from build123d import *

# Parameters (mm, degrees)
SKETCH_1_W               = 20
SKETCH_1_H               = 10
EXTRUDE_1_DEPTH          = 8.5
EXTRUDE_3_DEPTH          = 8.5
EXTRUDE_3_DEPTH_BACK     = 13
CUT_EXTRUDE_1_DEPTH      = 9
SKETCH_11_W              = 7.4
SKETCH_11_H              = 18
EXTRUDE_5_DEPTH          = 0.4
SKETCH_14_W              = 13
SKETCH_14_H              = 8.5
CUT_EXTRUDE_7_DEPTH      = 8
SKETCH_6_R               = 1.75
CUT_EXTRUDE_2_DEPTH      = 12.8
CUT_EXTRUDE_3_DEPTH      = 35.441980199
CUT_EXTRUDE_3_DEPTH_BACK = 12.9
SKETCH_15_W              = 3.5
SKETCH_15_H              = 8
CUT_EXTRUDE_8_DEPTH      = 8.5
SKETCH_12_R              = 1.6
CUT_EXTRUDE_4_DEPTH      = 35.693082884
SKETCH_13_R              = 3
CUT_EXTRUDE_5_DEPTH      = 4.5
FILLET_1_R               = 2.5
FILLET_2_R               = 4


# Some blends are built 0.0001 mm under size
with BuildPart() as part:
    # Эскиз1 → Бобышка-Вытянуть1 (new body)
    with BuildSketch(Plane.XY):
        with Locations((10, -5)):
            Rectangle(SKETCH_1_W, SKETCH_1_H)
    extrude(amount=EXTRUDE_1_DEPTH)

    # Эскиз4 → Бобышка-Вытянуть3 (add, two sides: drawn at the far end of the back side and taken through both)
    with BuildSketch(Plane(origin=(0, 0, 8.5), x_dir=(-1, 0, 0), z_dir=(0, 0, -1)).offset(-EXTRUDE_3_DEPTH_BACK)):
        with BuildLine():
            Line((4.25, -10), (0, -10))
            Line((0, -10), (0, 0))
            Line((0, 0), (-20, 0))
            Line((-20, 0), (-20, -10))
            Line((-20, -10), (-19.25, -10))
            Line((-19.25, -10), (-19.25, -14))
            ThreePointArc((-19.25, -14), (-18.078427125, -16.828427125), (-15.25, -18))
            Line((-15.25, -18), (4.25, -18))
            ThreePointArc((4.25, -18), (8.25, -14), (4.25, -10))
        make_face()
    extrude(amount=EXTRUDE_3_DEPTH + EXTRUDE_3_DEPTH_BACK)

    # Эскиз5 → Вырез-Вытянуть1 (cut)
    with BuildSketch(Plane.XY.offset(21.5)):
        Polygon((-1.25, -10), (-1.25, -18), (12.25, -18), (12.25, -10), (20, -10), (20, 0), (0, 0), (0, -10), align=None)
    extrude(amount=-CUT_EXTRUDE_1_DEPTH, mode=Mode.SUBTRACT)

    # Эскиз11 → Бобышка-Вытянуть5 (add)
    with BuildSketch(Plane(origin=(0, 0, 0), x_dir=(-1, 0, 0), z_dir=(0, 0, -1))):
        with Locations((-10, -9)):
            Rectangle(SKETCH_11_W, SKETCH_11_H)
    extrude(amount=EXTRUDE_5_DEPTH)

    # Эскиз14 → Вырез-Вытянуть7 (cut)
    with BuildSketch(Plane(origin=(9.75, -18, 0), x_dir=(-1, 0, 0), z_dir=(0, 1, 0))):
        with Locations((19.75, 4.25)):
            Rectangle(SKETCH_14_W, SKETCH_14_H)
    extrude(amount=CUT_EXTRUDE_7_DEPTH, mode=Mode.SUBTRACT)

    # Эскиз6 → Вырез-Вытянуть2 (cut)
    with BuildSketch(Plane.XY.offset(21.5)):
        with Locations((-4.25, -14)):
            Circle(SKETCH_6_R)
        with Locations((15.25, -14)):
            Circle(SKETCH_6_R)
    extrude(amount=-CUT_EXTRUDE_2_DEPTH, mode=Mode.SUBTRACT)

    # Эскиз7 → Вырез-Вытянуть3 (cut, two sides: drawn at the far end of the back side and taken through both)
    with BuildSketch(Plane(origin=(0, 0, 0), x_dir=(-1, 0, 0), z_dir=(0, 0, -1)).offset(-CUT_EXTRUDE_3_DEPTH_BACK)):
        Polygon((-15.25, -10.766838493), (-18.05, -12.383419246), (-18.05, -15.616580754), (-15.25, -17.233161507), (-12.45, -15.616580754), (-12.45, -12.383419246), align=None)
        Polygon((4.25, -10.766838493), (1.45, -12.383419246), (1.45, -15.616580754), (4.25, -17.233161507), (7.05, -15.616580754), (7.05, -12.383419246), align=None)
    extrude(amount=CUT_EXTRUDE_3_DEPTH + CUT_EXTRUDE_3_DEPTH_BACK, mode=Mode.SUBTRACT)

    # Эскиз15 → Вырез-Вытянуть8 (cut)
    with BuildSketch(Plane(origin=(0, 0, 0), x_dir=(-1, 0, 0), z_dir=(0, 0, -1))):
        with Locations((1.75, -14)):
            Rectangle(SKETCH_15_W, SKETCH_15_H)
    extrude(amount=-CUT_EXTRUDE_8_DEPTH, mode=Mode.SUBTRACT)

    # Эскиз12 → Вырез-Вытянуть4 (cut, through all)
    with BuildSketch(Plane(origin=(0, 0, -0.4), x_dir=(-1, 0, 0), z_dir=(0, 0, -1))):
        with Locations((-10, -5)):
            Circle(SKETCH_12_R)
    extrude(amount=-CUT_EXTRUDE_4_DEPTH, mode=Mode.SUBTRACT)

    # Эскиз13 → Вырез-Вытянуть5 (cut)
    with BuildSketch(Plane.XY.offset(12.5)):
        with Locations((10, -5)):
            Circle(SKETCH_13_R)
    extrude(amount=-CUT_EXTRUDE_5_DEPTH, mode=Mode.SUBTRACT)

    # Скругление1
    # the kernel refuses this fillet: 2.5 mm, written as the material it takes off along each edge
    with BuildSketch(Plane(origin=(0, 0, -6.25), x_dir=(1, 0, 0), z_dir=(0, 0, 1)), Plane(origin=(20, 0, 18.75), x_dir=(-1, 0, 0), z_dir=(0, 0, -1))) as fillet_1_piece_1:
        with BuildLine():
            CenterArc((FILLET_1_R, -FILLET_1_R), FILLET_1_R, 90, 90)
            Line((0, -FILLET_1_R), (-FILLET_1_R * 0.02, -FILLET_1_R))
            Line((-FILLET_1_R * 0.02, -FILLET_1_R), (-FILLET_1_R * 0.02, FILLET_1_R * 0.02))
            Line((-FILLET_1_R * 0.02, FILLET_1_R * 0.02), (FILLET_1_R, FILLET_1_R * 0.02))
            Line((FILLET_1_R, FILLET_1_R * 0.02), (FILLET_1_R, 0))
        make_face()
    extrude(amount=25, mode=Mode.SUBTRACT)
    with BuildSketch(Plane(origin=(20, -10, 16.963392768), x_dir=(0, 1, 0), z_dir=(0, 0, -1))) as fillet_1_piece_2:
        with BuildLine():
            CenterArc((1.785357107, -2.5), FILLET_1_R, 90, 45.572995999)
            Line((0, -0.75), (-0.035707142, -0.715))
            ThreePointArc((-0.035707142, -0.715), (-0.05, -0.375), (-0.05, 0))
            Line((-0.05, 0), (0, 0.05))
            Line((0, 0.05), (1.785357107, 0.05))
            Line((1.785357107, 0.05), (1.785357107, 0))
        make_face()
    extrude(amount=21.426785536, mode=Mode.SUBTRACT)

    # Скругление2
    fillet_2_edges = [part.edges().sort_by_distance(p)[0] for p in [
        (19.25, -10, 17),
    ]]
    fillet(fillet_2_edges, radius=FILLET_2_R - 0.0001)  # a hair under: the kernel refuses the full size


solid = part.part
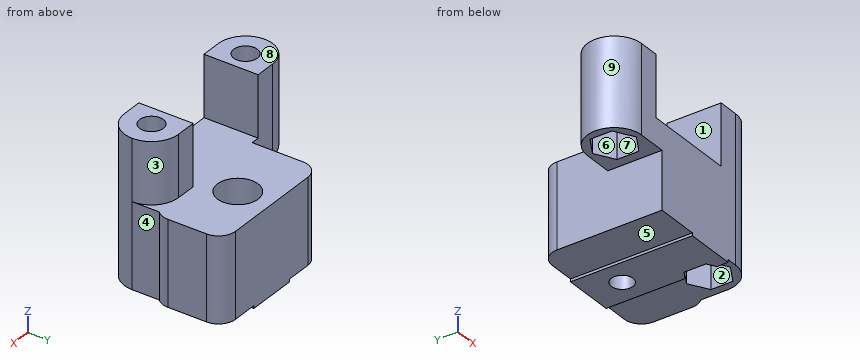
Read the model definition and answer for the solid it produces. Units are mm, in the model's axes. Face numbers are marked on the shaded views. A direction names the side the tool comes from. Coordinates: 2 decimals unless noted, no trailing zeros. Write each loop counter-clockwise with the first axis right and the second up, starting at its lowest first coordinate (ties: lowest second). Pieces come first, ordered by that corner, then holes. Notation, with made-up numbers: (56, 88) -> (94, 88) arc R19 cw to (94, 102) -> close; hole circle Ø1 at (-8, -12.75). An arc over 180 degrees is marked (long way). Return JSON: item names as keys, results as strings.
(1) The part is cut by section A-A on z = 17.25. State how many separate pieces and enclosed holes the cut face has, then the cut area to 3 significant figures.
Answers below:
{"separate pieces": "2", "enclosed holes": "2", "area": "79.0 mm^2"}
(2) The part is cut by section D-D on x = 10. Give the vertices of the cut face in (y, z), then the cut area to 3 significant figures.
Answers below:
{"outline": "(-18, -0.4) -> (-6.6, -0.4) -> (-6.6, 8) -> (-8, 8) -> (-8, 12.5) -> (-18, 12.5) -> close; (-3.4, -0.4) -> (0, -0.4) -> (0, 12.5) -> (-2, 12.5) -> (-2, 8) -> (-3.4, 8) -> close", "area": "178 mm^2"}
(3) Consider line 1 along Y through (x, z) = (15.25, 16.5); line 2 along Y through (x, z) = (10, 11.3); line 3 along X through (y, z) = (-15, 20.75). Determine where each line is inside the solid, lowest interval first. Write a range as from..to.
Answers below:
{"line 1": "-18..-15.75, -12.25..-10", "line 2": "-18..-8, -2..0", "line 3": "-8.12..-5.69, -2.81..-1.25, 12.25..13.81, 16.69..19.12"}
(4) Which of the six approach directions +Z, -Z, +X, -X, +Y, -Y give full straight-line access (tool end or side, diameter ignored) to the marked faces 1, 2, 3, 4 and 5?
Answers below:
{"face 1": "+Z, +Y, -Y", "face 2": "-Z", "face 3": "+Z, +X, +Y", "face 4": "+Z, -Z, +X, -Y", "face 5": "-Z, -X, +Y, -Y"}
(5) The part is cut by section B-B on y = -5. Give the vertices of the cut face in (x, z).
Answers below:
{"outline": "(0, 0) -> (6.3, 0) -> (6.3, -0.4) -> (8.4, -0.4) -> (8.4, 8) -> (7, 8) -> (7, 12.5) -> (0, 12.5) -> close; (11.6, -0.4) -> (13.7, -0.4) -> (13.7, 0) -> (20, 0) -> (20, 12.5) -> (13, 12.5) -> (13, 8) -> (11.6, 8) -> close"}
(6) The part is cut by section C-C on z = 6.75. Give the vertices of the cut face in (x, y).
Answers below:
{"outline": "(0, -18) -> (15.25, -18) arc R4 ccw to (19.25, -14) -> (19.25, -10) arc R2.5 ccw to (20, -8.21) -> (20, -2.5) arc R2.5 ccw to (17.5, 0) -> (2.5, 0) arc R2.5 ccw to (0, -2.5) -> close; hole circle Ø3.2 at (10, -5); hole (12.45, -15.62) -> (15.25, -17.23) -> (18.05, -15.62) -> (18.05, -12.38) -> (15.25, -10.77) -> (12.45, -12.38) -> close"}
(7) For a pull along Y with two mould halves and no side action, classify the marked faces 6, 7, 8 and 9 as pulls with the +Y half, pulls with the -Y half, needs draft (parallel to the pull), parting line crosses it, or undercut.
Answers below:
{"face 6": "undercut", "face 7": "undercut", "face 8": "needs draft", "face 9": "parting line crosses it"}
(8) Each of these flat-tipped pins is pushed along its axis until it touches: P1, Ø4, axis at x = 7.5, z = 7.5, coming from the +Y side; P2, Ø1, axis at y = -15, z = 12.5, coming from the +X side; P3, Ø10, axis at x = 7, y = -12, coming from the +Z side; P4, Ø4, axis at y = -14, z = 3, coming from the -X side. Where does it stop, or does it pass through?
Answers below:
{"P1": "y = 0", "P2": "x = 19.22", "P3": "z = 12.5", "P4": "x = 0"}
